Check sheet for the modelled part. Datum: model origin and axes. Units: mm. A direction names the side the tool comes from. Coordinates: 2 decimals unless noted, no trailing zeros. Loops run counter-clockwise (first coordinate to the right, second up) from the corner with the lowest first, then second, coordinate; pieces in that order, holes last. Notation, with made-up numbers: (31.5, 35.5) -> (83.5, 35.5) arc R30 ccw to (83.5, 57.5) -> close; hole circle Ø7 at (-30, 66.5). An arc over 180 degrees is marked (long way). Use CSV: the item, a comma, the result in double quotes.
```python
from build123d import *

# Parameters (mm, degrees)
SKETCH_1_W          = 25
SKETCH_1_H          = 30
EXTRUDE_2_DEPTH     = 18
CUT_EXTRUDE_1_DEPTH = 33
CUT_EXTRUDE_2_DEPTH = 33
SKETCH_6_R          = 3.5
CUT_EXTRUDE_3_DEPTH = 33
SKETCH_8_R          = 2
CUT_EXTRUDE_4_DEPTH = 6
FILLET_2_R          = 2


with BuildPart() as part:
    # 草图1 → 凸台-拉伸2 (new body)
    with BuildSketch(Plane(origin=(0, 0, 0), x_dir=(1, 0, 0), z_dir=(0, 1, 0))):
        with Locations((-18.558036971, -0.486406136)):
            Rectangle(SKETCH_1_W, SKETCH_1_H)
    extrude(amount=EXTRUDE_2_DEPTH)

    # 草图3 → 切除-拉伸1 (cut)
    with BuildSketch(Plane(origin=(-6.058036971, 0, 0), x_dir=(0, 0, -1), z_dir=(1, 0, 0))):
        Polygon((-15.486406136, 15), (-7.486406136, 15), (-4.486406136, 18), (-15.486406136, 18), align=None)
    extrude(amount=-CUT_EXTRUDE_1_DEPTH, mode=Mode.SUBTRACT)

    # 草图5 → 切除-拉伸2 (cut)
    with BuildSketch(Plane(origin=(-6.058036971, 0, 0), x_dir=(0, 0, -1), z_dir=(1, 0, 0))):
        Polygon((14.513593864, 18), (14.513593864, 15), (6.513593864, 15), (3.513593864, 18), align=None)
    extrude(amount=-CUT_EXTRUDE_2_DEPTH, mode=Mode.SUBTRACT)

    # 草图6 → 切除-拉伸3 (cut)
    with BuildSketch(Plane(origin=(-6.058036971, 0, 0), x_dir=(0, 0, -1), z_dir=(1, 0, 0))):
        with Locations((-0.486406136, 9)):
            Circle(SKETCH_6_R)
    extrude(amount=-CUT_EXTRUDE_3_DEPTH, mode=Mode.SUBTRACT)

    # 草图8 → 切除-拉伸4 (cut)
    with BuildSketch(Plane.XZ):
        with Locations(Location((-11.058036971, 10.486406136, 0), (0, 0, 270))):
            Circle(SKETCH_8_R)
        with Locations(Location((-11.058036971, -9.513593864, 0), (0, 0, 270))):
            Circle(SKETCH_8_R)
        with Locations(Location((-26.058036971, 10.486406136, 0), (0, 0, 270))):
            Circle(SKETCH_8_R)
        with Locations(Location((-26.058036971, -9.513593864, 0), (0, 0, 270))):
            Circle(SKETCH_8_R)
    extrude(amount=-CUT_EXTRUDE_4_DEPTH, mode=Mode.SUBTRACT)

    # 圆角2
    fillet_2_edges = [part.edges().sort_by_distance(p)[0] for p in [
        (-18.558036971, 18, 4.486406136),
        (-18.558036971, 15, 7.486406136),
        (-18.558036971, 15, 15.486406136),
        (-18.558036971, 18, -3.513593864),
        (-18.558036971, 15, -14.513593864),
        (-18.558036971, 15, -6.513593864),
        (-18.558036971, 0, -14.513593864),
        (-18.558036971, 0, 15.486406136),
    ]]
    fillet(fillet_2_edges, radius=FILLET_2_R)


solid = part.part
```
1) Cross-section at A-A on y = 9. Record the boundary of the cut face in (x, z).
Answer below:
outline,"(-31.06, -14.51) -> (-6.06, -14.51) -> (-6.06, -3.01) -> (-31.06, -3.01) -> close; (-31.06, 3.99) -> (-6.06, 3.99) -> (-6.06, 15.49) -> (-31.06, 15.49) -> close"
2) Access from +Z, -Z, +X, -X, +Y, -Y to the whole of each face (thin tool, end or side, straight path). Record for faces 1 (the cylindrical face through (-18.38, 0.57, -13.91)), 2 (the flat face through (-18, 15, -10)), 3 (the flat face through (-11, 6, -9)).
Answer below:
face 1,"-Z, +X, -X, -Y"
face 2,"-Z, +X, -X, +Y"
face 3,"-Y"
3) Thickness scan on line 1 along Y through (x, z) = (-24.5, 0.5); line 2 along Y through (x, z) = (-15, -11); line 3 along Z through (x, y) = (-28.75, 10.5). Record the ranges inside material, lowest first. Write a range as from..to.
Answer below:
line 1,"y = 0..5.5, 12.5..18"
line 2,"y = 0..15"
line 3,"z = -14.51..-2.68, 3.65..15.49"
4) Go/stop test with flat-tipped pins: pin 1 Ø3.5 at (x, z) = (-11.06, 10.49) entering from +Y; pin 2 Ø3 at (x, z) = (-26.06, 10.49) entering from -Y; pin 3 Ø6.5 at (x, z) = (-11.06, -9.51) entering from +Y. Record where each tip stops, or that it passes through.
Answer below:
pin 1,"stops at y = 15"
pin 2,"stops at y = 6"
pin 3,"stops at y = 15.32"
5) Cross-section at C-C on z = -1.75. Record the boundary of the cut face in (x, y), and give its area (3 significant figures).
Answer below:
outline,"(-31.06, 0) -> (-6.06, 0) -> (-6.06, 6.31) -> (-31.06, 6.31) -> close; (-31.06, 11.69) -> (-6.06, 11.69) -> (-6.06, 18) -> (-31.06, 18) -> close"
area,"315 mm²"
6) Draft check along X on faces 4 (the cylindrical face through (-26.824, 2.958, 8.639)), 5 (the flat face through (-19, 7, 15.486)), 6 (the flat face through (-31.058, 5, 1)). Enter one of: released by +X, released by -X, zero draft, split by the parting line, or undercut.
Answer below:
face 4,"undercut"
face 5,"zero draft"
face 6,"released by -X"
7) Cross-section at B-B on x = -22. Record the boundary of the cut face in (y, z).
Answer below:
outline,"(0, -12.51) arc R2 ccw to (2, -14.51) -> (13, -14.51) arc R2 ccw to (15, -12.51) -> (15, -7.34) arc R2 cw to (15.59, -5.93) -> (17.41, -4.1) arc R2 ccw to (18, -2.69) -> (18, 3.66) arc R2 ccw to (17.41, 5.07) -> (15.59, 6.9) arc R2 cw to (15, 8.31) -> (15, 13.49) arc R2 ccw to (13, 15.49) -> (2, 15.49) arc R2 ccw to (0, 13.49) -> close; hole circle Ø7 at (9, 0.49)"
8) Cross-section at D-D on y = 4.25. Record the boundary of the cut face in (x, z), and give its area (3 significant figures).
Answer below:
outline,"(-31.06, -14.51) -> (-6.06, -14.51) -> (-6.06, 15.49) -> (-31.06, 15.49) -> close; hole circle Ø4 at (-26.06, -9.51); hole circle Ø4 at (-26.06, 10.49); hole circle Ø4 at (-11.06, -9.51); hole circle Ø4 at (-11.06, 10.49)"
area,"700 mm²"
